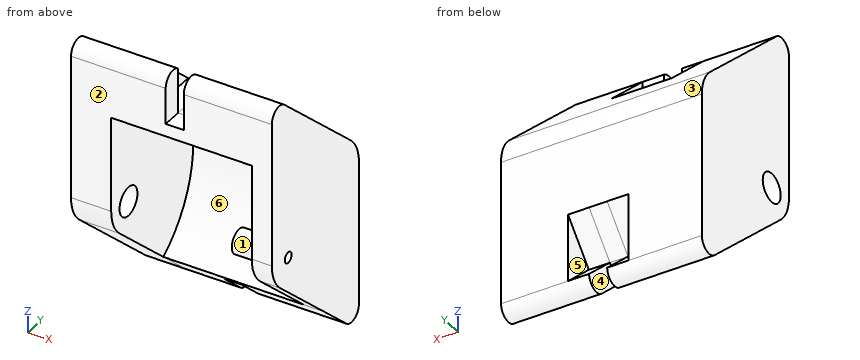
```python
from build123d import *

# Parameters (mm, degrees)
SKETCH4_R            = 3.6
THICKBASE_DEPTH      = 10
MIDDLE_DEPTH         = 35
THINBASE_DEPTH       = 5
SKETCH8_R            = 1.35
RETAINERSCREW_DEPTH  = 5
SKETCH9_R            = 3
SKETCH9_R_2          = 1.35
SPACER_DEPTH         = 7.2
SHOCKHOLE_START      = -35
SKETCH10_W           = 4.5
SKETCH10_H           = 12
SHOCKHOLE_DEPTH      = 17.524613
SKETCH12_W           = 15
SKETCH12_H           = 12.521275246
SHOCKHOLEBASE_DEPTH  = 82.308539587
SKETCH11_W           = 4.5
SKETCH11_H           = 12
SHOCKHOLE2_DEPTH     = 35
SKETCH13_W           = 15
SKETCH13_H           = 12.521275247
SHOCKHOLE2BASE_DEPTH = 80.489490329


with BuildPart() as part:
    # Sketch4 → ThickBase (new body)
    with BuildSketch(Plane(origin=(0, 0, 0), x_dir=(0, 0, -1), z_dir=(1, 0, 0))):
        with BuildLine():
            Line((-14.01318338, 16.550216151), (21.822267157, 16.550216151))
            ThreePointArc((21.822267157, 16.550216151), (24.561793845, 14.77291543), (24.055345362, 11.546878503))
            Line((24.055345362, 11.546878503), (0.125176293, -15.12757601))
            ThreePointArc((0.125176293, -15.12757601), (-3.242753458, -17.581539475), (-7.318417722, -18.449783849))
            Line((-7.318417722, -18.449783849), (-43.153868259, -18.449783849))
            ThreePointArc((-43.153868259, -18.449783849), (-45.893394947, -16.672483128), (-45.386946464, -13.446446201))
            Line((-45.386946464, -13.446446201), (-21.456777395, 13.228008312))
            ThreePointArc((-21.456777395, 13.228008312), (-18.088847644, 15.681971777), (-14.01318338, 16.550216151))
        make_face()
        with Locations((-5.952745457, -11.509649573)):
            Circle(SKETCH4_R, mode=Mode.SUBTRACT)
    extrude(amount=THICKBASE_DEPTH)

    # Sketch5 → Middle (add)
    with BuildSketch(Plane(origin=(10, 0, 0), x_dir=(0, 0, -1), z_dir=(1, 0, 0))):
        with BuildLine():
            Line((15.945305194, 2.506787856), (24.055345362, 11.546878503))
            ThreePointArc((24.055345362, 11.546878503), (24.561793845, 14.77291543), (21.822267157, 16.550216151))
            Line((21.822267157, 16.550216151), (-14.01318338, 16.550216151))
            ThreePointArc((-14.01318338, 16.550216151), (-18.088847644, 15.681971777), (-21.456777395, 13.228008312))
            Line((-21.456777395, 13.228008312), (-45.386946464, -13.446446201))
            ThreePointArc((-45.386946464, -13.446446201), (-45.893394947, -16.672483128), (-43.153868259, -18.449783849))
            Line((-43.153868259, -18.449783849), (-31.009075531, -18.449783849))
            ThreePointArc((-31.009075531, -18.449783849), (-16.549356077, 12.232654103), (15.945305194, 2.506787856))
        make_face()
    extrude(amount=MIDDLE_DEPTH)

    # Sketch7 → ThinBase (add)
    with BuildSketch(Plane(origin=(45, 0, 0), x_dir=(0, 0, -1), z_dir=(1, 0, 0))):
        with BuildLine():
            ThreePointArc((15.945305194, 2.506787856), (-16.549356077, 12.232654103), (-31.009075531, -18.449783849))
            Line((-31.009075531, -18.449783849), (-7.318417722, -18.449783849))
            ThreePointArc((-7.318417722, -18.449783849), (-3.242753458, -17.581539475), (0.125176293, -15.12757601))
            Line((0.125176293, -15.12757601), (15.945305194, 2.506787856))
        make_face()
        with BuildLine():
            Line((-43.153868259, -18.449783849), (-31.009075531, -18.449783849))
            ThreePointArc((-31.009075531, -18.449783849), (-16.549356077, 12.232654103), (15.945305194, 2.506787856))
            Line((15.945305194, 2.506787856), (24.055345362, 11.546878503))
            ThreePointArc((24.055345362, 11.546878503), (24.561793845, 14.77291543), (21.822267157, 16.550216151))
            Line((21.822267157, 16.550216151), (-14.01318338, 16.550216151))
            ThreePointArc((-14.01318338, 16.550216151), (-18.088847644, 15.681971777), (-21.456777395, 13.228008312))
            Line((-21.456777395, 13.228008312), (-45.386946464, -13.446446201))
            ThreePointArc((-45.386946464, -13.446446201), (-45.893394947, -16.672483128), (-43.153868259, -18.449783849))
        make_face()
    extrude(amount=THINBASE_DEPTH)

    # Sketch8 → RetainerScrew (cut)
    with BuildSketch(Plane(origin=(50, 0, 0), x_dir=(0, 0, -1), z_dir=(1, 0, 0))):
        with Locations((-5.789718886, -11.874919798)):
            Circle(SKETCH8_R)
    extrude(amount=-RETAINERSCREW_DEPTH, mode=Mode.SUBTRACT)

    # Sketch9 → Spacer (add)
    with BuildSketch(Plane.ZY.offset(-45)):
        with Locations(Location((5.789718886, -11.874919798, 0), (0, 0, 180))):
            Circle(SKETCH9_R)
        with Locations(Location((5.789718886, -11.874919798, 0), (0, 0, 180))):
            Circle(SKETCH9_R_2, mode=Mode.SUBTRACT)
    extrude(amount=SPACER_DEPTH)

    # Sketch10 → ShockHole (cut)
    with BuildSketch(Plane(origin=(0, 16.564225392, 18.463792524), x_dir=(1, 0, 0), z_dir=(0, 0.6677792161146302, 0.7443594014488768)).offset(SHOCKHOLE_START)):
        with Locations((25.82, 21.65868724)):
            Rectangle(SKETCH10_W, SKETCH10_H)
    extrude(amount=SHOCKHOLE_DEPTH, mode=Mode.SUBTRACT)

    # Sketch12 → ShockHoleBase (cut, through all)
    with BuildSketch(Plane(origin=(0, 11.655691061, -10.45654589), x_dir=(1, 0, 0), z_dir=(0, 0.7443594014488766, -0.6677792161146304))):
        with Locations((25.82, -1.068918271)):
            Rectangle(SKETCH12_W, SKETCH12_H)
    extrude(amount=SHOCKHOLEBASE_DEPTH, mode=Mode.SUBTRACT)

    # Sketch11 → ShockHole2 (cut)
    with BuildSketch(Plane(origin=(0, 16.550216151, 0), x_dir=(1, 0, 0), z_dir=(0, 1, 0))):
        with Locations((25.82, -40.153868259)):
            Rectangle(SKETCH11_W, SKETCH11_H)
    extrude(amount=-SHOCKHOLE2_DEPTH, mode=Mode.SUBTRACT)

    # Sketch13 → ShockHole2Base (cut, through all)
    with BuildSketch(Plane.XY.offset(34.153868259)):
        with Locations((25.82, -7.185808578)):
            Rectangle(SKETCH13_W, SKETCH13_H)
    extrude(amount=SHOCKHOLE2BASE_DEPTH, mode=Mode.SUBTRACT)


solid = part.part
```
The model under review builds one solid part; all positions refer to its coordinate system, in mm. Face numbers are marked on the shaded views. A direction names the side the tool comes from. Give positions to 0.01 mm unless a question says otherwise; leave off trailing zeros. Order: outer loops, then holes, each group sorted by start corner. A loop starts at its lowest first (then second) coordinate and runs counter-clockwise, first axis right, second up. Notation, with made-up numbers: (89.25, 80.5) - (106.25, 80.5) arc R17 cw to (106.25, 110.5) - close; hole circle Ø4 at (-20.5, 11.5). An arc over 180 degrees is marked (long way). Use CSV: the item, a comma, the result in double quotes. Start each with the question number.
Q1. To check wall thickness, follow line 1 along X through (y, z) = (-12, 11.5); line 2 along X through (y, z) = (11, -21); line 3 along Z through (x, y) = (10.5, 10.5). State the ranges of each line that lie inside material, in increasing order. Write a range as [from, to].
Q2. We need section B-B, the plane y = 10. Write out the cut boundary in (x, z), and give its area (3 significant figures).
Q3. The part is to be moulded in two halves that separate along Y. For the marked faces 1, 2 and 3, say which applies: +Y half, -Y half, draft (parallel to the pull), parting line (faces both ways), or undercut.
Q4. Tool access review of the marked faces 4, 5 and 6: name each direction out of +Z, -Z, +X, -X, +Y, -Y from which nothing blocks a thin tool from reaching the whole face with its end or side.
Q5. We need section D-D, the plane z = -2. Write out the cut boundary in (x, y).
Q6. Clearance check with flat-ended pins moving along their axes: pin 1 Ø10 at (x, y) = (23, 4.5) entering from -Z; pin 2 Ø6 at (x, z) = (29.5, 40) entering from +Y; pin 3 Ø6 at (x, y) = (31.5, -8.5) entering from +Z; pin 4 Ø2 at (y, z) = (-11.87, 5.79) entering from -X. State where each tip first meets the part, or that it passes through.
Q7. We need section A-A, the plane x = 42. Write out the cut boundary in (y, z).
Q8. We need section C-C, the plane x = 47.5. Write out the cut boundary in (y, z), and give its area (3 significant figures).
Outcome:
1,line 1,"x = [0, 10], [45, 50]"
1,line 2,"x = [0, 23.57], [28.07, 50]"
1,line 3,"z = [-23.12, -7.89], [19.79, 23.9]"
2,outline,"(0, -22.67) - (23.57, -22.67) - (23.57, -15.95) - (18.32, -15.95) - (18.32, -12.3) - (33.32, -12.3) - (33.32, -15.95) - (28.07, -15.95) - (28.07, -22.67) - (50, -22.67) - (50, 24.35) - (0, 24.35) - close; hole (10, -8.65) - (45, -8.65) - (45, 20.56) - (10, 20.56) - close"
2,area,"1,240 mm^2"
3,face 1,"undercut"
3,face 2,"-Y half"
3,face 3,"+Y half"
4,face 4,"-Z, +Y"
4,face 5,"+Y"
4,face 6,"none"
5,outline,"(0, -13.04) - (10, -13.04) - (10, 13.24) - (45, 13.24) - (45, -13.04) - (50, -13.04) - (50, 16.55) - (0, 16.55) - close"
6,pin 1,"stops at z = -22.22"
6,pin 2,"stops at y = -13.45"
6,pin 3,"stops at z = 43.09"
6,pin 4,"passes through"
7,outline,"(-18.45, 31.01) arc R26 cw to (2.51, -15.95) - (11.55, -24.06) arc R3 ccw to (16.55, -21.82) - (16.55, 14.01) arc R10 ccw to (13.23, 21.46) - (-13.45, 45.39) arc R3 ccw to (-18.45, 43.15) - close; circle Ø6 at (-11.87, 5.79); hole circle Ø2.7 at (-11.87, 5.79)"
8,outline,"(-18.45, 7.32) arc R10 ccw to (-15.13, -0.13) - (11.55, -24.06) arc R3 ccw to (16.55, -21.82) - (16.55, 14.01) arc R10 ccw to (13.23, 21.46) - (-13.45, 45.39) arc R3 ccw to (-18.45, 43.15) - close; hole circle Ø2.7 at (-11.87, 5.79)"
8,area,"1,620 mm^2"
